Check sheet for the modelled part. Datum: model origin and axes. Units: mm. Coordinates: 2 decimals unless noted, no trailing zeros. Order: outer loops, then holes, each group sorted by start corner. A loop starts at its lowest first (then second) coordinate and runs counter-clockwise, first axis right, second up. Notation, with made-up numbers: (-3, 66.25) -> (41, 66.25) arc R29 cw to (41, 99.25) -> close; hole circle Ø6 at (68.25, 61.5). An arc over 180 degrees is marked (long way). Put each result on its own line as item: value. Start each with the question number.
```python
from build123d import *

# Parameters (mm, degrees)
F1_DEPTH = 7
F2_R     = 2


with BuildPart() as f1:
    # F0 (on Top) → F1 (new body)
    with BuildSketch(Plane.XY):
        with BuildLine():
            ThreePointArc((-11, 0), (-7.7781745931, 7.7781745931), (0, 11))
            Line((0, 11), (-7.7157273072, 11))
            ThreePointArc((-7.7157273072, 11), (-11.9206288377, 6.1992786672), (-13.4362363733, 0))
            Line((-13.4362363733, 0), (-11, 0))
        make_face()
        with BuildLine():
            ThreePointArc((0, 11), (7.7781745931, 7.7781745931), (11, 0))
            Line((11, 0), (13.4362363733, 0))
            ThreePointArc((13.4362363733, 0), (11.9206288377, 6.1992786672), (7.7157273072, 11))
            Line((7.7157273072, 11), (0, 11))
        make_face()
        with BuildLine():
            Line((13.4362363733, 0), (11, 0))
            ThreePointArc((11, 0), (7.7781745931, -7.7781745931), (0, -11))
            Line((0, -11), (7.7157273072, -11))
            ThreePointArc((7.7157273072, -11), (11.9206288377, -6.1992786672), (13.4362363733, 0))
        make_face()
        with BuildLine():
            Line((7.7157273072, -11), (0, -11))
            Line((0, -11), (0, -13.4362363733))
            ThreePointArc((0, -13.4362363733), (4.0456055031, -12.8127094712), (7.7157273072, -11))
        make_face()
        with BuildLine():
            Line((0, -13.4362363733), (0, -11))
            Line((0, -11), (-7.7157273072, -11))
            ThreePointArc((-7.7157273072, -11), (-4.0456055031, -12.8127094712), (0, -13.4362363733))
        make_face()
        with BuildLine():
            Line((-7.7157273072, -11), (0, -11))
            ThreePointArc((0, -11), (-7.7781745931, -7.7781745931), (-11, 0))
            Line((-11, 0), (-13.4362363733, 0))
            ThreePointArc((-13.4362363733, 0), (-11.9206288377, -6.1992786672), (-7.7157273072, -11))
        make_face()
        with BuildLine():
            Line((-25.0909402017, -11), (-7.7157273072, -11))
            ThreePointArc((-7.7157273072, -11), (-11.9206288377, -6.1992786672), (-13.4362363733, 0))
            Line((-13.4362363733, 0), (-27.3962639826, 0))
            ThreePointArc((-27.3962639826, 0), (-26.8137399624, -5.619486581), (-25.0909402017, -11))
        make_face()
        with BuildLine():
            ThreePointArc((7.7157273072, 11), (11.9206288377, 6.1992786672), (13.4362363733, 0))
            Line((13.4362363733, 0), (27.3962639826, 0))
            ThreePointArc((27.3962639826, 0), (26.8137399624, 5.619486581), (25.0909402017, 11))
            Line((25.0909402017, 11), (7.7157273072, 11))
        make_face()
        with BuildLine():
            Line((0, 13.4362363733), (0, 11))
            Line((0, 11), (7.7157273072, 11))
            ThreePointArc((7.7157273072, 11), (4.0456055031, 12.8127094712), (0, 13.4362363733))
        make_face()
        with BuildLine():
            Line((-7.7157273072, 11), (0, 11))
            Line((0, 11), (0, 13.4362363733))
            ThreePointArc((0, 13.4362363733), (-4.0456055031, 12.8127094712), (-7.7157273072, 11))
        make_face()
        with BuildLine():
            Line((-23.8751509383, -13.4362363733), (0, -13.4362363733))
            ThreePointArc((0, -13.4362363733), (-4.0456055031, -12.8127094712), (-7.7157273072, -11))
            Line((-7.7157273072, -11), (-25.0909402017, -11))
            ThreePointArc((-25.0909402017, -11), (-24.5133296861, -12.2332312946), (-23.8751509383, -13.4362363733))
        make_face()
        with BuildLine():
            Line((23.8751509383, 13.4362363733), (0, 13.4362363733))
            ThreePointArc((0, 13.4362363733), (4.0456055031, 12.8127094712), (7.7157273072, 11))
            Line((7.7157273072, 11), (25.0909402017, 11))
            ThreePointArc((25.0909402017, 11), (24.5133296861, 12.2332312946), (23.8751509383, 13.4362363733))
        make_face()
    extrude(amount=F1_DEPTH)

    # F2
    f2_edges = [f1.edges().sort_by_distance(p)[0] for p in [
        (-9.500854, 9.500854, 7),
        (9.500854, -9.500854, 7),
        (-11.937575, -13.436236, 0),
        (-26.50137, -6.944975, 0),
        (11.937575, 13.436236, 0),
        (26.50137, 6.944975, 0),
        (20.41625, 0, 0),
        (-20.41625, 0, 0),
        (26.50137, 6.944975, 7),
        (-26.50137, -6.944975, 7),
        (20.41625, 0, 7),
        (-20.41625, 0, 7),
        (11.937575, 13.436236, 7),
    ]]
    fillet(f2_edges, radius=F2_R)


solid = f1.part
```
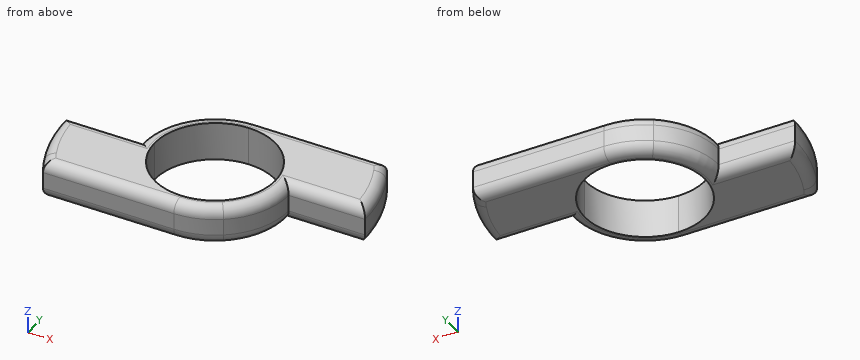
1) Gauge pin test, flat ends, axial feed: pin 1 (2 mm diameter, centred on y = -10.5, z = 4, fed in from +X); pin 2 (3.5 mm diameter, centred on x = 20, z = 3, fed in from -Y); pin 3 (2.5 mm diameter, centred on x = -20, z = 3.5, fed in from +Y). Record the tip position at first contact, or that the pin passes through.
2) Sectioned sample at B-B (x = 14). Record the boundary of the cut face in (y, z).
3) Sectioned sample at C-C (z = 5.75). Record the boundary of the cut face in (x, y), plus the area to 3 significant figures.
4) Scan lines: line 1 along X through (y, z) = (-0.5, 4.5); line 2 along Y through (x, z) = (-7, 3); line 3 along X through (y, z) = (7.5, 3.25). Record each from-to range of solid material in increasing order. Write a range as [from, to].
5) Sectioned sample at A-A (z = 2.75). Record the boundary of the cut face in (x, y), plus the area to 3 significant figures.
Entries:
1. pin 1: stops at x = 9.5
1. pin 2: stops at y = 0
1. pin 3: stops at y = 0
2. outline: (0, 2) arc R2 ccw to (2, 0) -> (11.44, 0) arc R2 ccw to (13.44, 2) -> (13.44, 5) arc R2 ccw to (11.44, 7) -> (2, 7) arc R2 ccw to (0, 5) -> close
3. outline: (-27.25, -0.15) arc R27.25 ccw to (-23.79, -13.29) -> (0, -13.29) arc R13.29 ccw to (13.29, 0.15) -> (27.25, 0.15) arc R27.25 ccw to (23.79, 13.29) -> (0, 13.29) arc R13.29 ccw to (-13.29, -0.15) -> close; hole circle Ø22 at (0, 0)
3. area: 588 mm2
4. line 1: x = [-27.39, -10.99], [10.99, 13.43]
4. line 2: y = [-13.44, -8.49], [8.49, 11.47]
4. line 3: x = [-11.15, -8.05], [8.05, 26.35]
5. outline: (-27.4, 0) arc R27.4 ccw to (-23.88, -13.44) -> (0, -13.44) arc R13.44 ccw to (13.44, 0) -> (27.4, 0) arc R27.4 ccw to (23.88, 13.44) -> (0, 13.44) arc R13.44 ccw to (-13.44, 0) -> close; hole circle Ø22 at (0, 0)
5. area: 609 mm2
